from build123d import *

# Parameters (mm, degrees)
BASPROSKE_W         = 4
BASPROSKE_H         = 21
TOOTHCUT_DEPTH      = 30.966648128
TEETHCUTS_COUNT     = 26
TEETHCUTS_ANGLE     = 346.153846154
BORSKE_R            = 3
BORE_DEPTH          = 50.0000508
EXTRUDE_START       = 11.5
EXTRUDE_1_DEPTH     = 11.5
SKETCH_2_R          = 1.25
CUT_EXTRUDE_1_DEPTH = 37.084686733


with BuildPart() as part:
    # BasProSke → Base-Revolve (revolve)
    with BuildSketch(Plane(origin=(0, 0, 0), x_dir=(1, 0, 0), z_dir=(0, 1, 0)), mode=Mode.PRIVATE) as base_revolve_sk:
        with Locations((2, 10.5)):
            Rectangle(BASPROSKE_W, BASPROSKE_H)
    revolve(base_revolve_sk.sketch.rotate(Axis((-10, 0, 0), (1, 0, 0)), 180), axis=Axis((-10, 0, 0), (1, 0, 0)))

    # TooCutSke → ToothCut (cut, through all)
    with BuildSketch(Plane(origin=(0, 0, 0), x_dir=(0, 0, -1), z_dir=(1, 0, 0))):
        with BuildLine():
            ThreePointArc((0.70920213, 17.609724823), (0, 17.624), (-0.70920213, 17.609724823))
            ThreePointArc((-0.70920213, 17.609724823), (-1.221230171, 19.346413175), (-2.119872395, 20.918259636))
            ThreePointArc((-2.119872395, 20.918259636), (0, 21.0254), (2.119872395, 20.918259636))
            ThreePointArc((2.119872395, 20.918259636), (1.221230171, 19.346413175), (0.70920213, 17.609724823))
        make_face()
    toothcut = extrude(amount=TOOTHCUT_DEPTH, mode=Mode.SUBTRACT)

    # TeethCuts: ToothCut ×26 about axis
    teethcuts_axis = Axis((-10, 0, 0), (1, 0, 0))
    for i in range(1, TEETHCUTS_COUNT):
        add(toothcut.rotate(teethcuts_axis, i * TEETHCUTS_ANGLE / (TEETHCUTS_COUNT - 1)), mode=Mode.SUBTRACT)

    # BorSke → Bore (cut, symmetric)
    with BuildSketch(Plane(origin=(0, 0, 0), x_dir=(0, 0, -1), z_dir=(1, 0, 0))):
        with Locations(Location((0, 0, 0), (0, 0, 180))):
            Circle(BORSKE_R)
    extrude(amount=BORE_DEPTH, both=True, mode=Mode.SUBTRACT)

    # 草图1 → 凸台-拉伸1 (add)
    with BuildSketch(Plane(origin=(4, 0, 0), x_dir=(0, 0, -1), z_dir=(1, 0, 0)).offset(EXTRUDE_START)):
        with BuildLine():
            Line((-4.005493963, 2.050857896), (-4.005493963, -2.050857896))
            ThreePointArc((-4.005493963, -2.050857896), (4.5, 0), (-4.005493963, 2.050857896))
        make_face()
        with BuildLine():
            Line((-2.505493963, 1.65), (-2.505493963, -1.65))
            ThreePointArc((-2.505493963, -1.65), (3, 0), (-2.505493963, 1.65))
        make_face(mode=Mode.SUBTRACT)
    extrude(amount=-EXTRUDE_1_DEPTH)

    # 草图2 → 切除-拉伸1 (cut, through all)
    with BuildSketch(Plane.XY.offset(4.005493963)):
        with Locations((13, 0)):
            Circle(SKETCH_2_R)
    extrude(amount=-CUT_EXTRUDE_1_DEPTH, mode=Mode.SUBTRACT)


solid = part.part
Read the model definition and answer for the solid it produces. Units are mm, in the model's axes. A direction names the side the tool comes from. Give positions to 0.01 mm unless a question says otherwise; leave off trailing zeros. Write each loop counter-clockwise with the first axis right and the second up, starting at its lowest first coordinate (ties: lowest second). Pieces come first, ordered by that corner, then holes. Notation, with made-up numbers: (71.5, 53.25) - (106.5, 53.25) arc R23 cw to (106.5, 70.25) - close; hole circle Ø8 at (64.5, 70.25). An arc over 180 degrees is marked (long way). Return JSON: item names as keys, results as strings.
Q1. Consider line 1 along Z through (x, y) = (8, 0); line 2 along Y through (x, z) = (2.3, 0); line 3 along X through (y, z) = (0.5, -6). Determine where each line is inside the solid, lowest interval first. Write a range as [from, to].
Reply:
{"line 1": "[-4.5, -3], [2.51, 4.01]", "line 2": "[-17.62, -3], [3, 17.62]", "line 3": "[0, 4]"}
Q2. A cutting plane is placed at A-A, the plane z = 0. Determine the outline of the cut face in (x, y).
Reply:
{"outline": "(0, -17.62) - (4, -17.62) - (4, -4.5) - (15.5, -4.5) - (15.5, -3) - (0, -3) - close; (0, 3) - (15.5, 3) - (15.5, 4.5) - (4, 4.5) - (4, 17.62) - (0, 17.62) - close"}
Q3. For a pull along Y with two mould halves and no side action, classify faces 5 (the face through (4, -5, 0)), 6 (the face through (1.97, -13.2, -11.68)), 7 (the face through (1.97, 1.13, 19.31)), 8 (the face through (1.97, 18.5, -5.82)) as released by +Y, released by -Y, zero draft, split by the parting line, or undercut.
Reply:
{"face 5": "zero draft", "face 6": "undercut", "face 7": "undercut", "face 8": "released by +Y"}
Q4. A cutting plane is placed at B-B, the plane x = 13. Determine the outline of the cut face in (y, z), and give its area (3 significant figures).
Reply:
{"outline": "(-2.05, 4.01) arc R4.5 ccw to (-1.25, -4.32) - (-1.25, -2.73) arc R3 cw to (-1.65, 2.51) - (-1.25, 2.51) - (-1.25, 4.01) - close; (1.25, -4.32) arc R4.5 ccw to (2.05, 4.01) - (1.25, 4.01) - (1.25, 2.51) - (1.65, 2.51) arc R3 cw to (1.25, -2.73) - close", "area": "27.5 mm²"}
Q5. Given P1, Ø5, axis at x = 9, z = -3.5, coming from the +Y side; P2, Ø1.6, axis at x = 7.5, y = 0.5, coming from the -Z side; P3, Ø4.5, axis at x = 12.5, y = 0, coming from the +Z side, each flat-ended and moving along its own axis, determine where each tip first touches the part or whether it passes through.
Reply:
{"P1": "y = 4.39", "P2": "z = -4.5", "P3": "z = 4.01"}
Q6. For faces 1 (the face through (2, 2.1, -17.5)), 2 (the face through (1.972, -7.975, 17.627)), 3 (the face through (1.972, 9.987, -16.626)), 4 (the face through (1.972, -19.356, 1.225)), determine the directions among +Z, -Z, +X, -X, +Y, -Y from which every point of the face is accessible in a straight line to the end or side of a thin tool.
Reply:
{"face 1": "-Z, +X, -X", "face 2": "+Z, +X, -X", "face 3": "+X, -X", "face 4": "+X, -X, -Y"}
Q7. A cutting plane is placed at C-C, the plane x = 10.25. Determine the outline of the cut face in (y, z).
Reply:
{"outline": "(-2.05, 4.01) arc R4.5 ccw (long way) to (2.05, 4.01) - close; hole (-1.65, 2.51) arc R3 ccw (long way) to (1.65, 2.51) - close"}
Q8. A cutting plane is placed at D-D, the plane y = 8.5. Determine the outline of the cut face in (x, z).
Reply:
{"outline": "(0, -18.13) - (4, -18.13) - (4, 18.13) - (0, 18.13) - close"}
